Design review of the part shown in the three views and the two pictorial views. Dimensions are in mm from the part's minimum x, y and z. Give positions to 0.01 mm unless a question says otherwise; leave off trailing zeros. Order: outer loops, then holes, each group sorted by start corner. A loop starts at its lowest first (then second) coordinate and runs counter-clockwise, first axis right, second up.
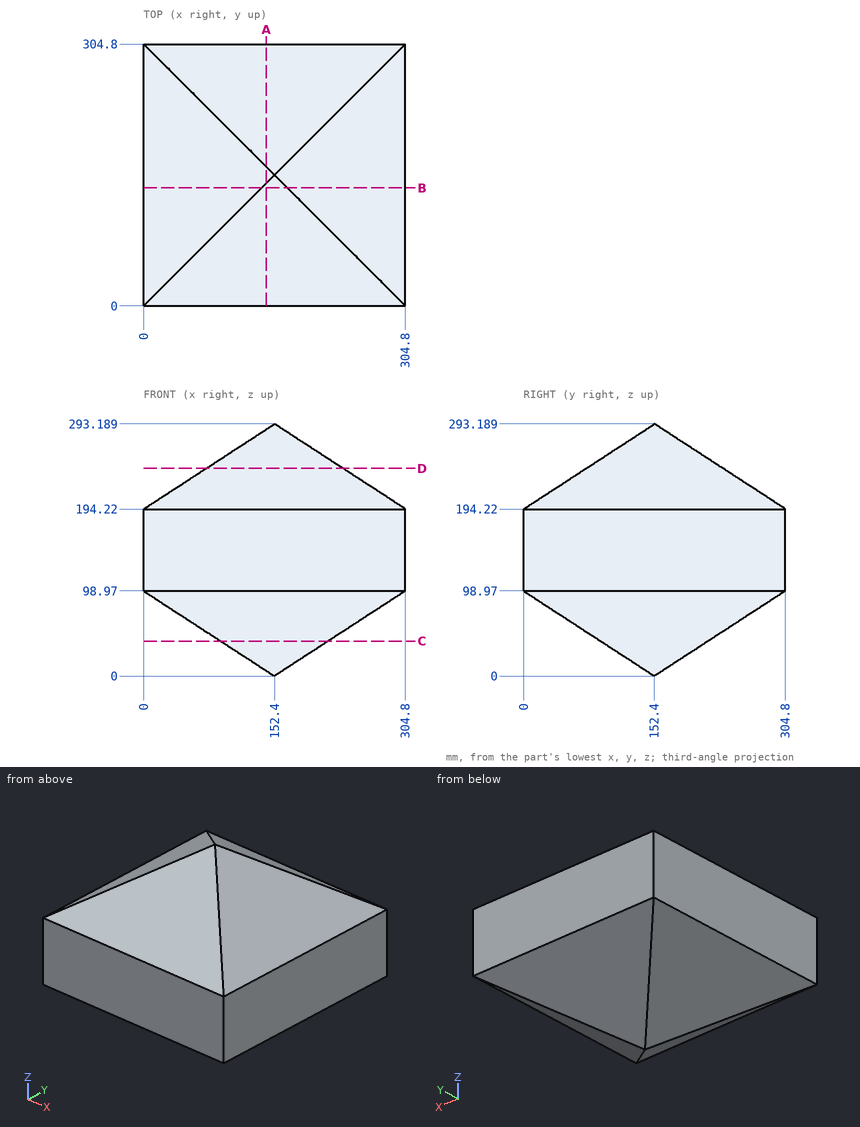
Item 1: Take a section at B-B (y = 137.5). Give the boundary of the cut face in (x, z), and give its area (3 significant figures).
Values found:
outline: (0, 98.97) - (137.5, 9.68) - (167.3, 9.68) - (304.8, 98.97) - (304.8, 194.22) - (167.3, 283.51) - (137.5, 283.51) - (0, 194.22) - close
area: 58,900 mm2
Item 2: Take a section at D-D (z = 241.5). Give the boundary of the cut face in (x, y) (1 decimal), and give its area (3 significant figures).
Values found:
outline: (72.8, 72.8) - (232, 72.8) - (232, 232) - (72.8, 232) - close
area: 25,300 mm2
Item 3: Clearance check with flat-ended pins moving along their axes: pin 1 Ø10 at (x, y) = (193.5, 186) entering from +Z (1 decimal); pin 2 Ø3 at (x, y) = (274, 205) entering from +Z (1 decimal); pin 3 Ø12 at (x, y) = (167, 240.5) entering from -Z. State where each tip first meets the part, or that it passes through.
Values found:
pin 1: stops at z = 269.7
pin 2: stops at z = 215.2
pin 3: stops at z = 53.32
Item 4: Take a section at C-C (z = 40.5). Give the boundary of the cut face in (x, y) (1 decimal).
Values found:
outline: (90, 90) - (214.8, 90) - (214.8, 214.8) - (90, 214.8) - close
Item 5: For line 1 (Z direction, x = 37.5, y = 165.5) (1 decimal); line 2 (Z direction, x = 109, y = 190.5) (1 decimal); line 3 (X direction, y = 205.5, z = 233) (1 decimal), list the stretches that pass through material, from the lowest coordinate up.
Values found:
line 1: z = 74.6 to 218.6
line 2: z = 28.2 to 265
line 3: x = 59.7 to 245.1
Item 6: Take a section at A-A (x = 143). Give the boundary of the cut face in (y, z) (1 decimal).
Values found:
outline: (0, 99) - (143, 6.1) - (161.8, 6.1) - (304.8, 99) - (304.8, 194.2) - (161.8, 287.1) - (143, 287.1) - (0, 194.2) - close
